The drawing under review shows one solid part. Ordinate dimensions are in mm from its lowest x, y, z. A direction names the side the tool comes from. Coordinates: 2 decimals unless noted, no trailing zeros. One line per item, written item: value. Start each with the question number.
1) Machinability: for the marked faces 4, 5 and 6, which of the approach directions +Z, -Z, +X, -X, +Y, -Y give a long, thin tool a straight path to every point of the face, cutting with its end or side? Answer none if there is none.
2) For probe 1 along Z at (x, y) = (34, 4.25) (1 decimal); probe 2 along Z at (x, y) = (29, 1.5) (1 decimal); probe 3 along X at (y, z) = (2.75, 18) (1 decimal), list the stretches that pass through material, from the lowest coordinate up. Write a range as from..to.
3) Mouldability with a two-part tool opening along Z and no side actions: class the marked faces 1, 2 and 3 as released by +Z, released by -Z, zero draft, split by the parting line, or undercut.
4) Add section C-C (y = 3.25). State how many separate pieces and enclosed holes the cut face has, and give its area (3 significant figures).
5) For pin 1 Ø3 at (x, y) = (5.5, 2.5) entering from +Z; pin 2 Ø1.5 at (x, y) = (16, 2) entering from -Z; pin 3 Ø1.9 at (y, z) = (2.5, 30.5) entering from -X; pin 4 Ø2 at (x, z) = (13.47, 22.45) entering from -Y, all flat-tipped, find the tip position at first contact; note any pin that passes through.
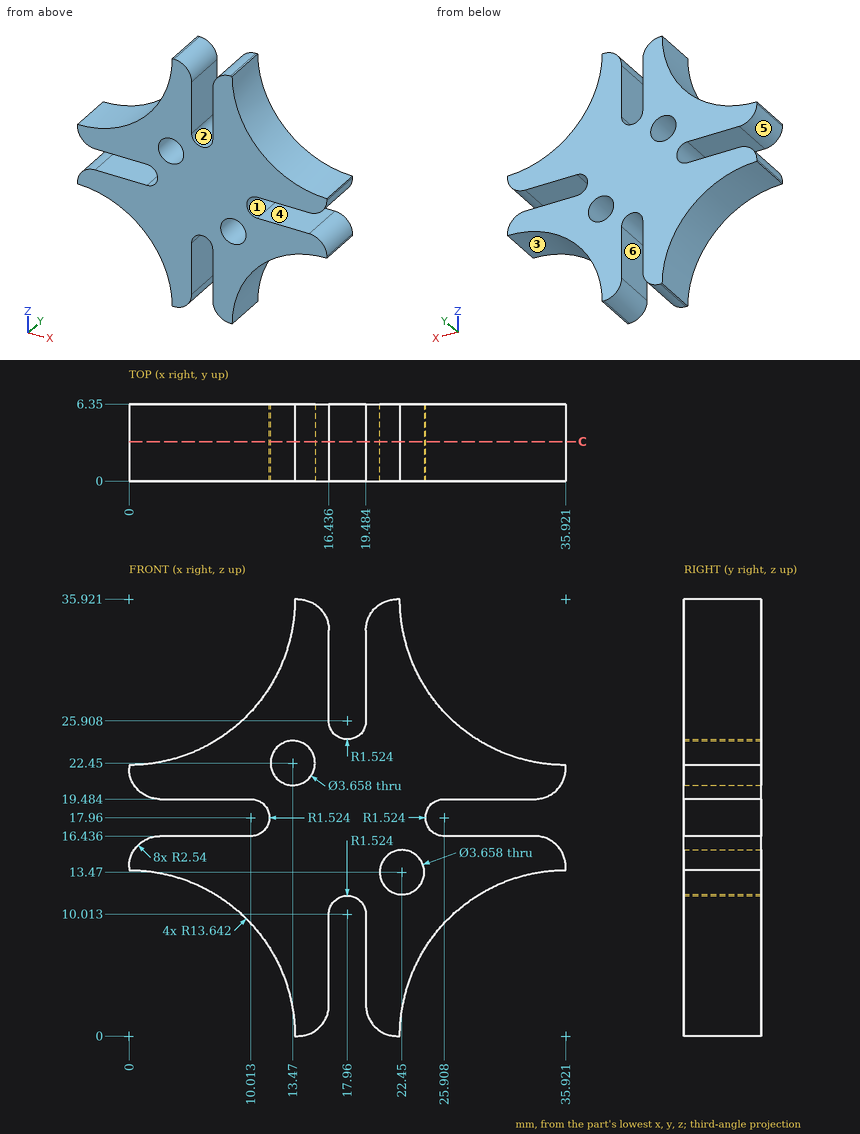
Numbers:
1. face 4: +X, +Y, -Y
1. face 5: -X, +Y, -Y
1. face 6: -Z, +Y, -Y
2. probe 1: 13.5..16.4, 19.6..22.4
2. probe 2: 11.8..16.4, 19.5..24.2
2. probe 3: 11.5..24.4
3. face 1: undercut
3. face 2: released by +Z
3. face 3: released by -Z
4. separate pieces: 1
4. enclosed holes: 2
4. area: 537 mm²
5. pin 1: z = 24.21
5. pin 2: z = 0.39
5. pin 3: x = 12.06
5. pin 4: through
